Answer from the drawing. Dimensions are ordinates in mm from the lowest x, y and z of the part. A direction names the side the tool comes from. Coordinates: 2 decimals unless noted, no trailing zeros. Write each loop counter-clockwise with the first axis right and the second up, starting at its lowest first coordinate (ties: lowest second). Pieces come first, ordered by that corner, then holes. Notation, with made-up numbers: M 13,55 L 68,55 A19 ccw 68,65 Z; hole C 43,-12.75 d7. An arc over 180 degrees is marked long. Put each result on its own line as item: value. Start each with the question number.
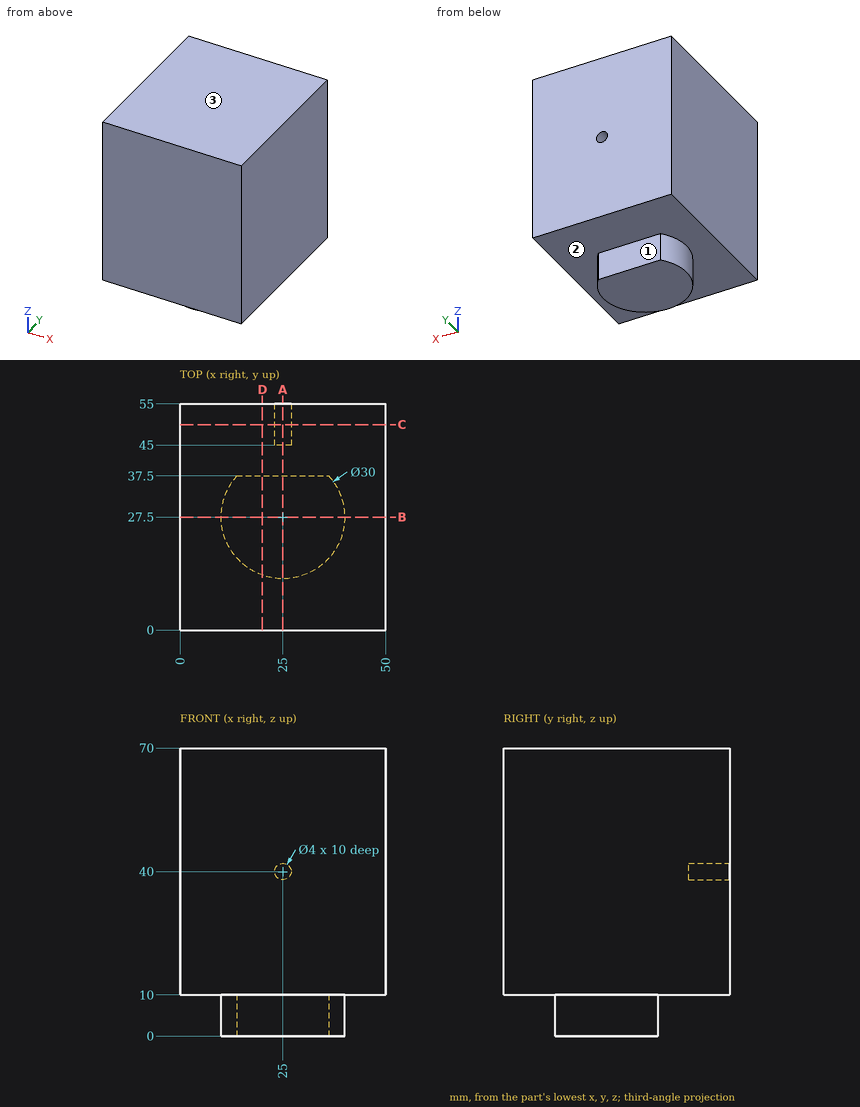
1) For the marked faces 1, 2 and 3, determine the directions among +Z, -Z, +X, -X, +Y, -Y from which every point of the face is accessible in a straight line to the end or side of a thin tool.
2) A cutting plane is placed at A-A on x = 25. Write down the section's boundary in (y, z).
3) A cutting plane is placed at B-B on y = 27.5. Write down the section's boundary in (x, z).
4) A cutting plane is placed at D-D on x = 20. Write down the section's boundary in (y, z).
5) Given pin 1 Ø5 at (x, y) = (21, 8.5) entering from -Z; pin 2 Ø5 at (x, z) = (27.5, 2.5) entering from +Y, each flat-ended and moving along its own axis, determine where each tip first touches the part or whether it passes through.
6) A cutting plane is placed at C-C on y = 50. Write down the section's boundary in (x, z).
7) Straight lines are drawn through the part: probe 1 along Z at (x, y) = (25, 49); probe 2 along Z at (x, y) = (43.5, 4); probe 3 along X at (y, z) = (50.25, 40). For each, find the intervals that lie inside material, in ascending order.
Answers follow:
1. face 1: -Z, +X, -X, +Y
1. face 2: -Z
1. face 3: +Z, +X, -X, +Y, -Y
2. outline: M 0,10 L 12.5,10 L 12.5,0 L 37.5,0 L 37.5,10 L 55,10 L 55,38 L 45,38 L 45,42 L 55,42 L 55,70 L 0,70 Z
3. outline: M 0,10 L 10,10 L 10,0 L 40,0 L 40,10 L 50,10 L 50,70 L 0,70 Z
4. outline: M 0,10 L 13.36,10 L 13.36,0 L 37.5,0 L 37.5,10 L 55,10 L 55,70 L 0,70 Z
5. pin 1: stops at z = 10
5. pin 2: stops at y = 37.5
6. outline: M 0,10 L 50,10 L 50,70 L 0,70 Z; hole C 25,40 d4
7. probe 1: z = 10 to 38, 42 to 70
7. probe 2: z = 10 to 70
7. probe 3: x = 0 to 23, 27 to 50
